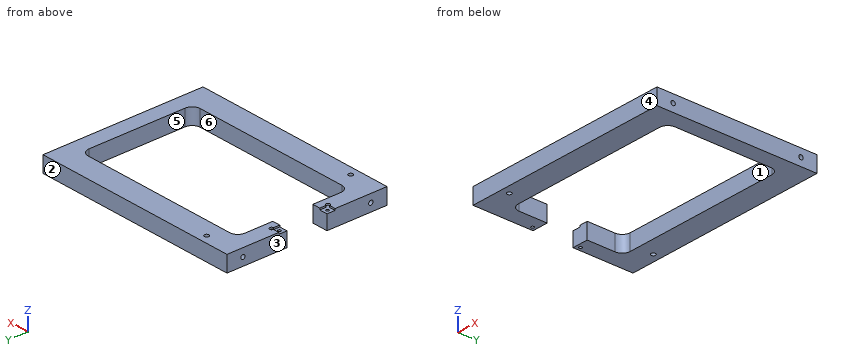
```python
from build123d import *

# Parameters (mm, degrees)
SKETCH1_W                 = 165.1
SKETCH1_H                 = 127
BOSS_EXTRUDE1_DEPTH       = 12.7
CUT_EXTRUDE1_DEPTH        = 105.919218926
SKETCH3_W                 = 6.477
SKETCH3_H                 = 6.477
CUT_EXTRUDE2_DEPTH        = 1.27
SKETCH4_W                 = 6.477
SKETCH4_H                 = 6.477
CUT_EXTRUDE3_DEPTH        = 1.27
F_8_32_TAPPED_HOLE1_D     = 3.4544
F_8_32_TAPPED_HOLE1_DEPTH = 12.7
F_8_32_TAPPED_HOLE1_TIP   = 1.037806461
F_8_32_TAPPED_HOLE2_D     = 3.4544
F_8_32_TAPPED_HOLE2_DEPTH = 12.7
F_8_32_TAPPED_HOLE2_TIP   = 1.037806461
F_8_32_TAPPED_HOLE3_D     = 3.4544
F_8_32_TAPPED_HOLE3_DEPTH = 12.7
F_8_32_TAPPED_HOLE3_TIP   = 1.037806461
F_8_32_TAPPED_HOLE4_D     = 3.4544
F_8_32_TAPPED_HOLE4_DEPTH = 12.7
F_8_32_TAPPED_HOLE4_TIP   = 1.037806461
F_4_40_TAPPED_HOLE1_D     = 2.2606
F_4_40_TAPPED_HOLE2_D     = 2.2606
SKETCH20_R                = 1.778
CUT_EXTRUDE4_DEPTH        = 105.919218926
SKETCH21_R                = 1.778
CUT_EXTRUDE5_DEPTH        = 105.919218926
FILLET4_R                 = 6.35
FILLET5_R                 = 6.35
SKETCH24_R                = 1.5875
CUT_EXTRUDE6_DEPTH        = 1.27


with BuildPart() as part:
    # Sketch1 → Boss-Extrude1 (new body)
    with BuildSketch(Plane.XY):
        Rectangle(SKETCH1_W, SKETCH1_H)
    extrude(amount=BOSS_EXTRUDE1_DEPTH)

    # Sketch2 → Cut-Extrude1 (cut, through all)
    with BuildSketch(Plane.XY):
        Polygon((-82.55, -15.875), (-69.85, -15.875), (-69.85, -44.45), (69.85, -44.45), (69.85, 44.45), (-69.85, 44.45), (-69.85, 15.875), (-82.55, 15.875), align=None)
    extrude(amount=CUT_EXTRUDE1_DEPTH, mode=Mode.SUBTRACT)

    # Sketch3 → Cut-Extrude2 (cut)
    with BuildSketch(Plane.XY.offset(12.7)):
        with Locations((-79.3115, 19.1135)):
            Rectangle(SKETCH3_W, SKETCH3_H)
    extrude(amount=-CUT_EXTRUDE2_DEPTH, mode=Mode.SUBTRACT)

    # Sketch4 → Cut-Extrude3 (cut)
    with BuildSketch(Plane.XY.offset(12.7)):
        with Locations((-79.3115, -19.1135)):
            Rectangle(SKETCH4_W, SKETCH4_H)
    extrude(amount=-CUT_EXTRUDE3_DEPTH, mode=Mode.SUBTRACT)

    # #8-32 Tapped Hole1
    with Locations(Plane.ZY.offset(82.55)):
        with Locations((6.35, 50.8)):
            Hole(F_8_32_TAPPED_HOLE1_D / 2, depth=F_8_32_TAPPED_HOLE1_DEPTH)
            with Locations((0, 0, -(F_8_32_TAPPED_HOLE1_DEPTH + F_8_32_TAPPED_HOLE1_TIP / 2))):  # 118° drill point
                Cone(0, F_8_32_TAPPED_HOLE1_D / 2, F_8_32_TAPPED_HOLE1_TIP, mode=Mode.SUBTRACT)

    # #8-32 Tapped Hole2
    with Locations(Plane.ZY.offset(82.55)):
        with Locations((6.35, -50.689875403)):
            Hole(F_8_32_TAPPED_HOLE2_D / 2, depth=F_8_32_TAPPED_HOLE2_DEPTH)
            with Locations((0, 0, -(F_8_32_TAPPED_HOLE2_DEPTH + F_8_32_TAPPED_HOLE2_TIP / 2))):  # 118° drill point
                Cone(0, F_8_32_TAPPED_HOLE2_D / 2, F_8_32_TAPPED_HOLE2_TIP, mode=Mode.SUBTRACT)

    # #8-32 Tapped Hole3
    with Locations(Plane(origin=(82.55, 0, 0), x_dir=(0, 0, -1), z_dir=(1, 0, 0))):
        with Locations((-6.35, 50.8)):
            Hole(F_8_32_TAPPED_HOLE3_D / 2, depth=F_8_32_TAPPED_HOLE3_DEPTH)
            with Locations((0, 0, -(F_8_32_TAPPED_HOLE3_DEPTH + F_8_32_TAPPED_HOLE3_TIP / 2))):  # 118° drill point
                Cone(0, F_8_32_TAPPED_HOLE3_D / 2, F_8_32_TAPPED_HOLE3_TIP, mode=Mode.SUBTRACT)

    # #8-32 Tapped Hole4
    with Locations(Plane(origin=(82.55, 0, 0), x_dir=(0, 0, -1), z_dir=(1, 0, 0))):
        with Locations((-6.35, -50.689875403)):
            Hole(F_8_32_TAPPED_HOLE4_D / 2, depth=F_8_32_TAPPED_HOLE4_DEPTH)
            with Locations((0, 0, -(F_8_32_TAPPED_HOLE4_DEPTH + F_8_32_TAPPED_HOLE4_TIP / 2))):  # 118° drill point
                Cone(0, F_8_32_TAPPED_HOLE4_D / 2, F_8_32_TAPPED_HOLE4_TIP, mode=Mode.SUBTRACT)

    # #4-40 Tapped Hole1 (through all)
    with Locations(Plane.XY.offset(11.43)):
        with Locations((-79.375, 19.05)):
            Hole(F_4_40_TAPPED_HOLE1_D / 2)

    # #4-40 Tapped Hole2 (through all)
    with Locations(Plane.XY.offset(11.43)):
        with Locations((-79.375, -19.05)):
            Hole(F_4_40_TAPPED_HOLE2_D / 2)

    # Sketch20 → Cut-Extrude4 (cut, through all)
    with BuildSketch(Plane.XY.offset(12.7)):
        with Locations((-57.15, -57.15)):
            Circle(SKETCH20_R)
    extrude(amount=-CUT_EXTRUDE4_DEPTH, mode=Mode.SUBTRACT)

    # Sketch21 → Cut-Extrude5 (cut, through all)
    with BuildSketch(Plane.XY.offset(12.7)):
        with Locations((-57.15, 57.15)):
            Circle(SKETCH21_R)
    extrude(amount=-CUT_EXTRUDE5_DEPTH, mode=Mode.SUBTRACT)

    # Fillet4
    fillet4_edges = [part.edges().sort_by_distance(p)[0] for p in [
        (-69.85, -44.45, 6.35),
    ]]
    fillet(fillet4_edges, radius=FILLET4_R)

    # Fillet5
    fillet5_edges = [part.edges().sort_by_distance(p)[0] for p in [
        (69.85, -44.45, 6.35),
        (69.85, 44.45, 6.35),
        (-69.85, 44.45, 6.35),
    ]]
    fillet(fillet5_edges, radius=FILLET5_R)

    # Sketch24 → Cut-Extrude6 (cut)
    with BuildSketch(Plane.XY.offset(12.7)):
        with Locations((-76.073, -22.352)):
            Circle(SKETCH24_R)
        with Locations((-76.073, 22.352)):
            Circle(SKETCH24_R)
    extrude(amount=-CUT_EXTRUDE6_DEPTH, mode=Mode.SUBTRACT)


solid = part.part
```
For this review, take the finished solid that the model builds, in its own axes (mm). Face numbers are marked on the shaded views. A direction names the side the tool comes from. Coordinates: 2 decimals unless noted, no trailing zeros. Write each loop counter-clockwise with the first axis right and the second up, starting at its lowest first coordinate (ties: lowest second). Pieces come first, ordered by that corner, then holes. Notation, with made-up numbers: (22.5, -39.75) - (60.5, -39.75) arc R10 ccw to (60.5, -35.75) - close; hole circle Ø10 at (31, -39). An arc over 180 degrees is marked (long way). Put each result on its own line as item: value.
1. Add section B-B, the plane y = -27. Give the boundary of the cut face in (x, z), then the cut area to 3 significant figures.
Values found:
outline: (-82.55, 0) - (-69.85, 0) - (-69.85, 12.7) - (-82.55, 12.7) - close; (69.85, 0) - (82.55, 0) - (82.55, 12.7) - (69.85, 12.7) - close
area: 323 mm²
2. Add section A-A, the plane x = -57.15. Give the boundary of the cut face in (y, z).
Values found:
outline: (-63.5, 0) - (-58.93, 0) - (-58.93, 12.7) - (-63.5, 12.7) - close; (-55.37, 0) - (-44.45, 0) - (-44.45, 12.7) - (-55.37, 12.7) - close; (44.45, 0) - (55.37, 0) - (55.37, 12.7) - (44.45, 12.7) - close; (58.93, 0) - (63.5, 0) - (63.5, 12.7) - (58.93, 12.7) - close
3. Wall thickness on probe 1 along Y at (x, z) = (78, 6.35); probe 2 along X at (y, z) = (17.5, 9.25); probe 3 along Y at (x, z) = (12.5, 7.25): over which ranges is each line inside the solid? List them lowest first.
Values found:
probe 1: -63.5 to -52.42, -48.96 to 49.07, 52.53 to 63.5
probe 2: -82.55 to -69.85, 69.85 to 82.55
probe 3: -63.5 to -44.45, 44.45 to 63.5
4. Add section C-C, the plane z = 9.75. Give the boundary of the cut face in (x, y) (3 decimals), then the cut area to 3 significant figures.
Values found:
outline: (-82.55, -63.5) - (82.55, -63.5) - (82.55, 63.5) - (-82.55, 63.5) - (-82.55, 15.875) - (-69.85, 15.875) - (-69.85, 38.1) arc R6.35 cw to (-63.5, 44.45) - (63.5, 44.45) arc R6.35 cw to (69.85, 38.1) - (69.85, -38.1) arc R6.35 cw to (63.5, -44.45) - (-63.5, -44.45) arc R6.35 cw to (-69.85, -38.1) - (-69.85, -15.875) - (-82.55, -15.875) - close; hole circle Ø2.261 at (-79.375, -19.05); hole circle Ø2.261 at (-79.375, 19.05); hole circle Ø3.556 at (-57.15, -57.15); hole circle Ø3.556 at (-57.15, 57.15)
area: 8,150 mm²
5. For pin 1 (3 mm diameter, centred on y = 50.8, z = 6.35, fed in from -X); pin 2 (6 mm diameter, centred on y = 7, z = 9.5, fed in from -X), all flat-tipped, find the tip position at first contact; note any pin that passes through.
Values found:
pin 1: x = -69.71
pin 2: x = 69.85
6. Machinability: for the marked faces 1 and 2, which of the approach directions +Z, -Z, +X, -X, +Y, -Y give a long, thin tool a straight path to every point of the face, cutting with its end or side? Answer none if there is none.
Values found:
face 1: +Z, -Z
face 2: +Z, -Z, +X, -X, +Y
7. Add section D-D, the plane x = 4.5. Give the boundary of the cut face in (y, z), then the cut area to 3 significant figures.
Values found:
outline: (-63.5, 0) - (-44.45, 0) - (-44.45, 12.7) - (-63.5, 12.7) - close; (44.45, 0) - (63.5, 0) - (63.5, 12.7) - (44.45, 12.7) - close
area: 484 mm²
8. Mouldability with a two-part tool opening along Y and no side actions: class the marked faces 3, 4, 5 and 6 as released by +Y, released by -Y, zero draft, split by the parting line, or undercut.
Values found:
face 3: zero draft
face 4: released by -Y
face 5: undercut
face 6: undercut
